Part model, mm, in its own coordinate system. Coordinates: 2 decimals unless noted, no trailing zeros. Loops run counter-clockwise (first coordinate to the right, second up) from the corner with the lowest first, then second, coordinate; pieces in that order, holes last. Notation, with made-up numbers: M 80.5,8 L 136.5,8 A28 ccw 136.5,34 Z; hole C 64,-32 d2. An arc over 180 degrees is marked long. Use CSV: the item, a comma, the result in double quotes. Start each with the question number.
from build123d import *

# Parameters (mm, degrees)
F0_R     = 11.2
F1_DEPTH = 7


with BuildPart() as f1:
    # F0 (on Top) → F1 (new body)
    with BuildSketch(Plane.XY):
        with BuildLine():
            ThreePointArc((1.78587, 52.038384), (0.064532, 52.918286), (-1.704408, 52.138489))
            Line((-1.704408, 52.138489), (-19.066227, 22.201317))
            ThreePointArc((-19.066227, 22.201317), (-15.219751, 8.713844), (-28.836632, 5.354102))
            Line((-28.836632, 5.354102), (-45.811212, -23.915348))
            ThreePointArc((-45.811212, -23.915348), (-45.706618, -26.395442), (-43.605451, -27.717147))
            Line((-43.605451, -27.717147), (-9.689672, -27.717147))
            ThreePointArc((-9.689672, -27.717147), (0.044547, -17.537595), (9.778766, -27.717147))
            Line((9.778766, -27.717147), (44.043854, -27.717147))
            ThreePointArc((44.043854, -27.717147), (46.3259, -26.513132), (46.431202, -23.935091))
            Line((46.431202, -23.935091), (29.068287, 5.61158))
            ThreePointArc((29.068287, 5.61158), (15.203422, 8.742665), (19.215132, 22.378807))
            Line((19.215132, 22.378807), (1.78587, 52.038384))
        make_face()
        with Locations((-24.390228, -14.081704)):
            Circle(F0_R, mode=Mode.SUBTRACT)
        Circle(F0_R, mode=Mode.SUBTRACT)
        with Locations((24.390229, -14.081704)):
            Circle(F0_R, mode=Mode.SUBTRACT)
        with Locations((0, 28.163411)):
            Circle(F0_R, mode=Mode.SUBTRACT)
    extrude(amount=F1_DEPTH)


solid = f1.part
1. Pin check, flat tips, straight feed: pin 1 (4 mm diameter, centred on x = 1.5, z = 2.5, fed in from -Y); pin 2 (4 mm diameter, centred on y = 11, z = 1.5, fed in from -X). Stop position of each tip, or through.
2. Wall check: probe 1 along Y at (x, z) = (0, 5.25); probe 2 along Y at (x, z) = (-8, 6); probe 3 along X at (y, z) = (-5, 0.5). Give the ranges that are in metal, low to high.
3. Slice it at A-A, the plane x = -24.5. List the corners of the cut face in (y, z), and give its area (3 significant figures).
4. Slice it at B-B, the plane y = -20.5. List the corners of the cut face in (x, z).
5. Slice it at C-C, the plane x = 18. List the corners of the cut face in (y, z).
6. Slice it at D-D, the plane z = 3. List the corners of the cut face in (x, y).
7. Two-plate mould, pull along X, no slides. Class faces 1 (the face through (-2.43, 17.23, 3.45)), 2 (the face through (-27, -27.717, 3)), 3 (the face through (37.87, -9.37, 3.45)): pulls with the +X half, pulls with the -X half, needs draft (parallel to the pull), parting line crosses it, or undercut.
Found:
1,pin 1,"y = -18.17"
1,pin 2,"x = -15.06"
2,probe 1,"-17.54 to -11.2, 11.2 to 16.96, 39.36 to 52.92"
2,probe 2,"-21.78 to -7.84, 7.84 to 20.33, 36 to 41.28"
2,probe 3,"-34.84 to -30.94, -17.84 to -10.02, 10.02 to 17.84, 30.94 to 35.3"
3,outline,"M -27.72,0 L -25.28,0 L -25.28,7 L -27.72,7 Z; M -2.88,0 L 3.9,0 L 3.9,7 L -2.88,7 Z"
3,area,"64.5 mm^2"
4,outline,"M -43.83,0 L -33.57,0 L -33.57,7 L -43.83,7 Z; M -15.21,0 L -6.95,0 L -6.95,7 L -15.21,7 Z; M 7.04,0 L 15.21,0 L 15.21,7 L 7.04,7 Z; M 33.57,0 L 44.41,0 L 44.41,7 L 33.57,7 Z"
5,outline,"M -27.72,0 L -23.28,0 L -23.28,7 L -27.72,7 Z; M -4.88,0 L 5.71,0 L 5.71,7 L -4.88,7 Z; M 21.65,0 L 24.45,0 L 24.45,7 L 21.65,7 Z"
6,outline,"M -45.81,-23.92 A2.67 ccw -43.61,-27.72 L -9.69,-27.72 A9.74 cw long 9.78,-27.72 L 44.04,-27.72 A2.59 ccw 46.43,-23.94 L 29.07,5.61 A9.74 cw long 19.22,22.38 L 1.79,52.04 A2.25 ccw -1.7,52.14 L -19.07,22.2 A9.74 cw long -28.84,5.35 Z; hole C -24.39,-14.08 d22.4; hole C 0,0 d22.4; hole C 0,28.16 d22.4; hole C 24.39,-14.08 d22.4"
7,face 1,"undercut"
7,face 2,"needs draft"
7,face 3,"pulls with the +X half"
